from build123d import *

# Parameters (mm, degrees)
SKETCH1_R           = 5
SKETCH1_R_2         = 2.5
BOSS_EXTRUDE1_DEPTH = 3.175
SKETCH2_R           = 4.75
SKETCH2_R_2         = 2.75
CUT_EXTRUDE1_DEPTH  = 2


with BuildPart() as part:
    # Sketch1 → Boss-Extrude1 (new body)
    with BuildSketch(Plane(origin=(0, 0, 0), x_dir=(1, 0, 0), z_dir=(0, 1, 0))):
        Circle(SKETCH1_R)
        Circle(SKETCH1_R_2, mode=Mode.SUBTRACT)
    extrude(amount=BOSS_EXTRUDE1_DEPTH)

    # Sketch2 → Cut-Extrude1 (cut)
    with BuildSketch(Plane(origin=(0, 3.175, 0), x_dir=(1, 0, 0), z_dir=(0, 1, 0))):
        Circle(SKETCH2_R)
        Circle(SKETCH2_R_2, mode=Mode.SUBTRACT)
    extrude(amount=-CUT_EXTRUDE1_DEPTH, mode=Mode.SUBTRACT)


solid = part.part
Model file for the job. Use its own axes, mm. Coordinates: 2 decimals unless noted, no trailing zeros. Order: outer loops, then holes, each group sorted by start corner. A loop starts at its lowest first (then second) coordinate and runs counter-clockwise, first axis right, second up. Notation, with made-up numbers: M 37.5,59.25 L 71.5,59.25 A18 ccw 71.5,63.25 Z; hole C 7.25,-37 d8. An arc over 180 degrees is marked long. Return JSON: item names as keys, results as strings.
1. Saw through at D-D (z = -4.5). Give the cut face in (x, y) (3 decimals), and give its area (3 significant figures).
Ans:
{"outline": "M -2.179,0 L 2.179,0 L 2.179,3.175 L 1.521,3.175 L 1.521,1.175 L -1.521,1.175 L -1.521,3.175 L -2.179,3.175 Z", "area": "7.76 mm^2"}
2. Saw through at B-B (z = 0). Give the cut face in (x, y) (3 decimals).
Ans:
{"outline": "M -5,0 L -2.5,0 L -2.5,3.175 L -2.75,3.175 L -2.75,1.175 L -4.75,1.175 L -4.75,3.175 L -5,3.175 Z; M 2.5,0 L 5,0 L 5,3.175 L 4.75,3.175 L 4.75,1.175 L 2.75,1.175 L 2.75,3.175 L 2.5,3.175 Z"}
3. Saw through at A-A (x = 0). Give the cut face in (y, z) (3 decimals), and give its area (4 significant figures).
Ans:
{"outline": "M 0,-5 L 3.175,-5 L 3.175,-4.75 L 1.175,-4.75 L 1.175,-2.75 L 3.175,-2.75 L 3.175,-2.5 L 0,-2.5 Z; M 0,2.5 L 3.175,2.5 L 3.175,2.75 L 1.175,2.75 L 1.175,4.75 L 3.175,4.75 L 3.175,5 L 0,5 Z", "area": "7.875 mm^2"}
4. Flat gauge pins, fed straight in: pin 1 (3 mm diameter, centred on x = 0.5, z = -1.5, fed in from +Y) (3 decimals); pin 2 (1 mm diameter, centred on y = 1.5, z = 1, fed in from +X); pin 3 (4.5 mm diameter, centred on x = 0, z = 0, fed in from +Y). Where does each tip first touch, or does it go through?
Ans:
{"pin 1": "y = 3.175", "pin 2": "x = 4.97", "pin 3": "through"}
5. Saw through at C-C (y = 2.55). Give the cut face in (x, z).
Ans:
{"outline": "C 0,0 d10; C 0,0 d5.5; hole C 0,0 d9.5; hole C 0,0 d5"}
6. Pull direction X, two halves, no side cores. Call faces 1 (the face through (-1.08, 1.57, 4.88)), 2 (the face through (2, 0, 2)), 3 (the face through (-0.54, 1.57, 2.44)): +X half, -X half, draft (parallel to the pull), parting line (faces both ways), or undercut.
Ans:
{"face 1": "parting line", "face 2": "draft", "face 3": "undercut"}
7. Drill centre lines: probe 1 along Z at (x, y) = (0, 1.8); probe 2 along Z at (x, y) = (-1.25, 2.2). Where is each one in solid material? Low to high.
Ans:
{"probe 1": "-5 to -4.75, -2.75 to -2.5, 2.5 to 2.75, 4.75 to 5", "probe 2": "-4.84 to -4.58, -2.45 to -2.17, 2.17 to 2.45, 4.58 to 4.84"}
